Work out the finished part from the listing and answer in its coordinate system (mm). Face numbers are marked on the shaded views. A direction names the side the tool comes from. Coordinates: 2 decimals unless noted, no trailing zeros. Order: outer loops, then holes, each group sorted by start corner. A loop starts at its lowest first (then second) coordinate and runs counter-clockwise, first axis right, second up. Notation, with made-up numbers: M -6,-35.5 L 34,-35.5 A12 cw 34,-23.5 Z; hole C -2,15.25 d8. An arc over 180 degrees is marked long. Answer in a Markdown table with one row per item. Add a question column.
Item 1: The part is cut by section C-C (z = -79). Write down the section's boundary in (x, y), then the cut area to 3 significant figures.
Item 2: Which of the six approach directions +Z, -Z, +X, -X, +Y, -Y give full straight-line access (tool end or side, diameter ignored) to the marked faces 1 and 2?
Item 3: The part is cut by section D-D (y = -5). Write down the section's boundary in (x, z), then the cut area to 3 significant figures.
Item 4: The part is cut by section A-A (x = 0). Write down the section's boundary in (y, z), then the cut area to 3 significant figures.
Item 5: Consider line 1 (X direction, y = 0, z = -77.25); line 2 (X direction, y = 0, z = -68.75); line 3 (Z direction, x = 0.5, y = 18). Determine where each line is inside the solid, lowest interval first. Write a range as from..to.
Item 6: Flat-ended cylindrical pins translate along their axes: pin 1 Ø8 at (y, z) = (-17.5, -77) entering from -X; pin 2 Ø8 at (x, y) = (15.5, 11) entering from -Z; pin 3 Ø2 at (x, z) = (0, -79) entering from +Y. Find the tip coordinate at first contact, or state that the pin passes through.
Item 7: The mould has two halves that part along Y. Classify the marked faces 3, 4 and 5: released by +Y, released by -Y, zero draft, split by the parting line, or undercut.
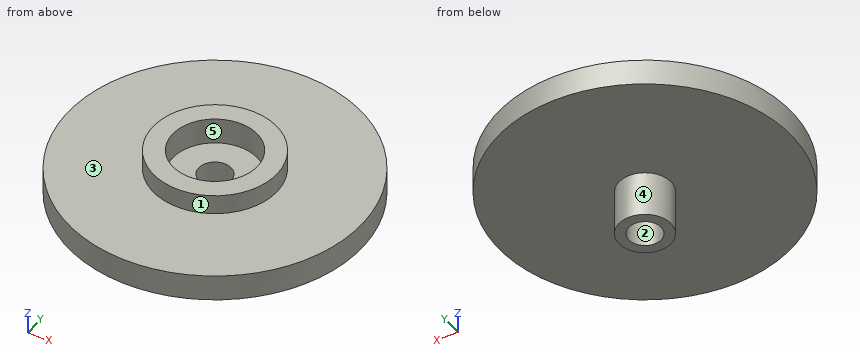
Autodesk Inventor part; units mm, degrees
ref_plane "YZ Plane" through (0, 0, 0) normal (1, 0, 0) x (0, 1, 0)
ref_plane "XZ Plane" through (0, 0, 0) normal (0, 1, 0) x (-1, 0, 0)
ref_plane "XY Plane" through (0, 0, 0) normal (0, 0, 1) x (1, 0, 0)
sketch "Sketch1" plane through (0, 0, 0) normal (1, 0, 0) x (0, 1, 0)
  line L0 (0, 0) -> (2.5, 0)
  line L1 (0, 0) -> (4, 0)
  line L2 (2.5, 0) -> (2.5, -7)
  line L3 (2.5, -7) -> (0, -7)
  line L4 (0, -7) -> (20, -7)
  line L5 (4, 0) -> (4, -7)
  line L6 (2.5, -7) -> (2.5, -41)
  line L7 (20, -7) -> (20, -11)
  line L8 (20, -11) -> (2.5, -11)
  line L9 (20, -7) -> (22.5, -7)
  line L10 (22.5, -7) -> (22.5, -11)
  line L11 (22.5, -11) -> (20, -11)
  line L12 (20, -11) -> (20, -7)
  line L13 (20, -7) -> (20, -11)
  line L14 (4, 0) -> (2.5, 0)
  line L15 (2.5, 0) -> (2.5, -11)
  line L16 (2.5, -11) -> (4, -11)
  line L17 (4, -11) -> (4, 0)
  line L18 (2.5, -11) -> (22.5, -11)
  line L19 (22.5, -11) -> (22.5, -7)
  line L20 (22.5, -7) -> (2.5, -7)
  line L21 (2.5, -7) -> (2.5, -11)
  line L22 (2.5, -11) -> (6.5, -11)
  line L23 (0, -7) -> (0, -105.9451)
  line L24 (2.5, -41) -> (25, -41)
  line L25 (0, -82) -> (2.5, -82)
  line L26 (0, -82) -> (4, -82)
  line L27 (2.5, -82) -> (2.5, -75)
  line L28 (2.5, -75) -> (0, -75)
  line L29 (0, -75) -> (20, -75)
  line L30 (4, -82) -> (4, -75)
  line L31 (20, -75) -> (20, -71)
  line L32 (20, -71) -> (2.5, -71)
  line L33 (20, -75) -> (22.5, -75)
  line L34 (22.5, -75) -> (22.5, -71)
  line L35 (22.5, -71) -> (20, -71)
  line L36 (20, -71) -> (20, -75)
  line L37 (20, -75) -> (20, -71)
  line L38 (4, -82) -> (2.5, -82)
  line L39 (2.5, -82) -> (2.5, -71)
  line L40 (2.5, -71) -> (4, -71)
  line L41 (4, -71) -> (4, -82)
  line L42 (2.5, -71) -> (22.5, -71)
  line L43 (22.5, -71) -> (22.5, -75)
  line L44 (22.5, -75) -> (2.5, -75)
  line L45 (2.5, -75) -> (2.5, -71)
  line L46 (2.5, -71) -> (6.5, -71)
  line L47 (2.5, -11) -> (6.5, -11)
  line L48 (6.5, -11) -> (6.5, -71)
  line L49 (6.5, -71) -> (2.5, -71)
  line L50 (2.5, -71) -> (2.5, -11)
  line L51 (6.5, -11) -> (9.5, -11)
  line L52 (9.5, -11) -> (9.5, -14)
  line L53 (9.5, -14) -> (6.5, -14)
  line L54 (6.5, -14) -> (6.5, -11)
  line L55 (6.5, -71) -> (9.5, -71)
  line L56 (9.5, -71) -> (9.5, -68)
  line L57 (9.5, -68) -> (6.5, -68)
  line L58 (6.5, -68) -> (6.5, -71)
  dimension "d1" = 2.5
  dimension "d2" = 4
  dimension "d3" = 7
  dimension "d4" = 20
  dimension "d5" = 34
  dimension "d9" = 4
  dimension "d12" = 2.5
  dimension "d13" = 4
  dimension "d55" = 22.5
  dimension "d56" = 4
  dimension "d80" = 3
  dimension "d81" = 3
  dimension "d82" = 3
  dimension "d83" = 3
revolve "Revolution2" add sketch "Sketch1" angle 360 about axis through (0, 0, -7) along (0, 0, -1) contours L1 L5 L4 L2 | L4 L17 L8 L6 | L4 L7 L8 L17 | L8 L48 L24 L6 | L9 L10 L11 L7 | L24 L48 L32 L50 | L8 L52 L53 L48 | L29 L30 L26 L27 | L39 L32 L41 L29 | L41 L32 L31 L29 | L57 L56 L32 L48 | L31 L35 L34 L33
sketch "Sketch6" plane through (0, 0, 0) normal (0, 1, 0) x (-1, 0, 0)
  line L0 (-2.5, -82) -> (2.5, -82)
  line L1 (0, -82) -> (0, -62)
  line L2 (0, -82) -> (20, -82) construction
  line L3 (0, -65) -> (15, -65) construction
  line L4 (0, -59) -> (15, -59) construction
  line L5 (10.6066, -48.3934) -> (10.6066, -54.3934)
  line L6 (0, -65) -> (0, -59)
  line L7 (0, -62) -> (0, -59.5)
  line L8 (0, -59.5) -> (10.6066, -48.8934)
  line L9 (10.6066, -48.8934) -> (10.6066, -53.8934)
  line L10 (10.6066, -53.8934) -> (0, -64.5)
  line L11 (0, -59.5) -> (0, -64.5)
  point P0 (0, 0)
  dimension "d64" = 20
  dimension "d65" = 90
  dimension "d69" = 15
  dimension "d71" = 15
  dimension "d75" = 2.5
  dimension "d76" = 5
extrude "Extrusion6" cut sketch "Sketch6" along normal mid plane 5
sketch "Sketch7" plane through (0, 0, 0) normal (0, 0, 1) x (1, 0, 0)
  arc A0 (-1.9966, -1.5104) -> (-1.9966, 1.4896) centre (0.0034, -0.0104) ccw
  line L0 (-1.9966, -0.0104) -> (-1.9966, 1.4896)
  line L1 (-1.9966, -0.0104) -> (-1.9966, -1.5104)
  line L2 (-1.9966, 1.4896) -> (-1.9966, -2.007)
  line L3 (-1.9966, -2.007) -> (-3.9862, -2.007)
  line L4 (-3.9862, -2.007) -> (-3.9862, 1.4896)
  line L5 (-3.9862, 1.4896) -> (-1.9966, 1.4896)
  line L6 (-1.9966, -1.5104) -> (-3.2272, -1.5104)
  line L7 (-3.2272, -1.5104) -> (-3.2272, 1.4896)
  line L8 (-3.2272, 1.4896) -> (-1.9966, 1.4896)
  line L9 (-1.9966, 1.4896) -> (-1.9966, -1.5104)
  point P0 (0, 0)
  point P1 (0, 0)
  dimension "d77" = 5
extrude "Extrusion7" add sketch "Sketch7" against normal blind 26 contours L6 L7 L5 L0 L1
sketch "Sketch8" plane through (0, 0, -68) normal (0, 0, 1) x (1, 0, 0)
  arc A0 (0, 2.5) -> (0, -2.5) centre (0, 0) ccw
  circle A1 centre (0, 0) radius 6.5
  point P0 (0, 0)
extrude "Extrusion8" cut sketch "Sketch8" against normal blind 4
sketch "Sketch9" plane through (0, 0, -68) normal (0, 0, 1) x (1, 0, 0)
  circle A0 centre (0, 0) radius 2.5
  circle A1 centre (0, 0) radius 22.5
  point P0 (0, 0)
extrude "Extrusion9" cut sketch "Sketch9" along normal blind 100 contours A0 | A1
properties part number "Spool_revB1"
Reply:
| question | item | result |
|---|---|---|
| 1 | outline | C 0,0 d8; hole C 0,0 d5 |
| 1 | area | 30.6 mm2 |
| 2 | face 1 | +Z |
| 2 | face 2 | +Z, -Z |
| 3 | outline | M -21.94,-75 L 21.94,-75 L 21.94,-71 L 8.08,-71 L 8.08,-68 L 4.15,-68 L 4.15,-72 L -4.15,-72 L -4.15,-68 L -8.08,-68 L -8.08,-71 L -21.94,-71 Z |
| 3 | area | 191 mm2 |
| 4 | outline | M -22.5,-75 L -4,-75 L -4,-82 L -2.5,-82 L -2.5,-72 L -6.5,-72 L -6.5,-68 L -9.5,-68 L -9.5,-71 L -22.5,-71 Z; M 2.5,-82 L 4,-82 L 4,-75 L 22.5,-75 L 22.5,-71 L 9.5,-71 L 9.5,-68 L 6.5,-68 L 6.5,-72 L 2.5,-72 Z |
| 4 | area | 191 mm2 |
| 5 | line 1 | x = -4..-2.5, 2.5..4 |
| 5 | line 2 | x = -9.5..-6.5, 6.5..9.5 |
| 5 | line 3 | z = -75..-71 |
| 6 | pin 1 | stops at x = -17.59 |
| 6 | pin 2 | stops at z = -75 |
| 6 | pin 3 | stops at y = 4 |
| 7 | face 3 | zero draft |
| 7 | face 4 | split by the parting line |
| 7 | face 5 | undercut |
